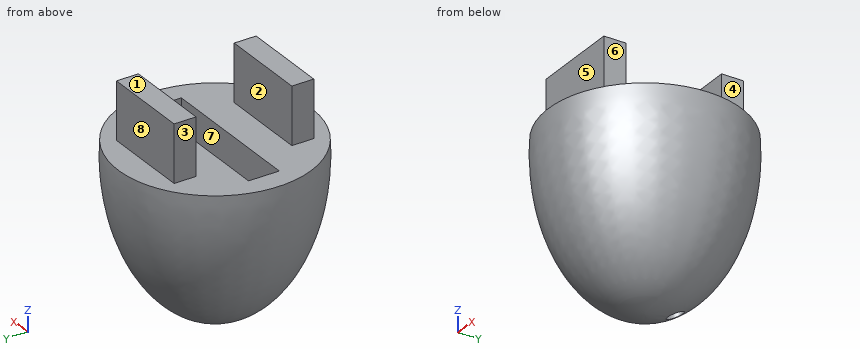
Autodesk Inventor part; units mm, degrees
ref_plane "YZ Plane" through (0, 0, 0) normal (1, 0, 0) x (0, 1, 0)
ref_plane "XZ Plane" through (0, 0, 0) normal (0, 1, 0) x (-1, 0, 0)
ref_plane "XY Plane" through (0, 0, 0) normal (0, 0, 1) x (1, 0, 0)
sketch "Sketch1" plane through (0, 0, 0) normal (0, 1, 0) x (-1, 0, 0)
  ellipse E0 centre (0, 0) end of major axis (0, 17.78) minor radius 11.2075
  line L0 (11.1609, 1.6196) -> (-11.1609, 1.6196)
  line L1 (0, -17.78) -> (0, 1.6196)
  line L2 (8.595, 11.4106) -> (-8.6719, 11.4106)
  dimension "d0" = 17.78
  dimension "d11" = 9.7909
  dimension "d16" = 19.3997
revolve "Revolution1" add sketch "Sketch1" angle 360 about axis through (0, 0, -17.78) along (0, 0, 1) picked at (-2.3015, -10.0552) contours L0 L1 E0
sketch "Sketch2" plane through (0, 0, 1.6196) normal (0, 0, 1) x (1, 0, 0)
  line L0 (-8.636, 1.778) -> (8.636, 1.778)
  line L1 (8.636, 1.778) -> (8.636, -1.778)
  line L2 (8.636, -1.778) -> (-8.636, -1.778)
  line L3 (-8.636, -1.778) -> (-8.636, 1.778)
  line L4 (-8.636, 1.778) -> (8.636, -1.778) construction
  line L5 (8.636, 1.778) -> (-8.636, -1.778) construction
  point P0 (0, 0)
  dimension "d2" = 17.272
  dimension "d3" = 3.556
extrude "Extrusion1" cut sketch "Sketch2" against normal blind 10.16
sketch "Sketch3" plane through (0, 0, 1.6196) normal (0, 0, 1) x (1, 0, 0)
  line L0 (-5.11, 8.0772) -> (5.05, 8.0772)
  line L1 (5.05, 8.0772) -> (5.05, 5.5372)
  line L2 (5.05, 5.5372) -> (-5.11, 5.5372)
  line L3 (-5.11, 5.5372) -> (-5.11, 8.0772)
  line L4 (-5.11, 8.0772) -> (5.05, 5.5372) construction
  line L5 (5.05, 8.0772) -> (-5.11, 5.5372) construction
  circle A0 centre (0, 0) radius 11.1609
  line L6 (-11.1609, 0) -> (11.1609, 0)
  line L7 (11.2075, 0) -> (0, 0)
  line L8 (-5.11, -8.0772) -> (5.05, -8.0772)
  line L9 (5.05, -8.0772) -> (5.05, -5.5372)
  line L10 (5.05, -5.5372) -> (-5.11, -5.5372)
  line L11 (-5.11, -5.5372) -> (-5.11, -8.0772)
  point P0 (-0.03, 6.8072)
  dimension "d6" = 10.16
  dimension "d7" = 2.54
  dimension "d12" = 6.8072
extrude "Extrusion2" add sketch "Sketch3" along normal blind 6.604 contours L0 L1 L2 L3 | L11 L10 L9 L8
sketch "Sketch4" plane through (0, 0, 1.6196) normal (0, 0, 1) x (1, 0, 0)
  circle A0 centre (0, 3.497) radius 0.889
  point P0 (0, 0)
  dimension "d13" = 1.778
extrude "Extrusion3" cut sketch "Sketch4" against normal through all
properties part number "Bead Round Button copy 1"
Geometry: final body of the model. Coordinates: model frame, mm. Face numbers are marked on the shaded views. A direction names the side the tool comes from. Give positions to 0.01 mm unless a question says otherwise; leave off trailing zeros. Order: outer loops, then holes, each group sorted by start corner. A loop starts at its lowest first (then second) coordinate and runs counter-clockwise, first axis right, second up. Notation, with made-up numbers: M 59.25,65 L 111.25,65 A24 ccw 111.25,96 Z; hole C 86,51.25 d2. An arc over 180 degrees is marked long. Answer as CSV lines item,"result". Start each with the question number.
1) Line query: line 1 (Y direction, x = 0, z = -2.25); line 2 (Y direction, x = 0, z = -5.5); line 3 (Y direction, x = 3, z = 1.75). Output: solid intervals per line, ascending. Write a range as from..to.
2) Set-up query: the marked faces 1, 2, 3 and 4. Return all of +Z, -Z, +X, -X, +Y, -Y with unobstructed straight access to the full face (end or side cutting, diameter ignored); none if empty.
3) Mould query, pull axis Y, two halves, no side actions, for the marked faces 5, 6, 7 and 8. Classes: +Y half, -Y half, draft (parallel to the pull), parting line (faces both ways), or undercut.
4) Cut plane B-B (z = -7.75). State how many separate pieces and enclosed holes the cut face has, then the cut area to 3 significant figures.
5) Cut plane A-A (z = 4.75). Output: boundary loops of the cut face in (x, y), then the cut area to 3 significant figures.
6) First-contact query: P1, Ø6, axis at x = -3, y = -1.5, coming from the +Z side; P2, Ø11, axis at x = -3.5, z = -4, coming from the +Y side; P3, Ø1.3, axis at y = -7, z = 6.5, coming from the -X side; P4, Ø0.8, axis at y = -6.5, z = 4.5, coming from the +X side. Flat tips, straight axial feed; report the tip coordinate or a pass-through.
Findings below:
1,line 1,"y = -11.12..-1.78, 1.78..2.61, 4.39..11.12"
1,line 2,"y = -10.66..-1.78, 1.78..2.61, 4.39..10.66"
1,line 3,"y = -8.08..-5.54, 5.54..8.08"
2,face 1,"+Z, +X, -X, +Y, -Y"
2,face 2,"+Z, +X, -X"
2,face 3,"+Z, -X, +Y, -Y"
2,face 4,"+Z, +X, +Y, -Y"
3,face 5,"-Y half"
3,face 6,"draft"
3,face 7,"undercut"
3,face 8,"+Y half"
4,separate pieces,"1"
4,enclosed holes,"2"
4,area,"256 mm²"
5,outline,"M -5.11,-8.08 L 5.05,-8.08 L 5.05,-5.54 L -5.11,-5.54 Z; M -5.11,5.54 L 5.05,5.54 L 5.05,8.08 L -5.11,8.08 Z"
5,area,"51.6 mm²"
6,P1,"stops at z = 1.62"
6,P2,"stops at y = 11.21"
6,P3,"stops at x = -5.11"
6,P4,"stops at x = 5.05"
